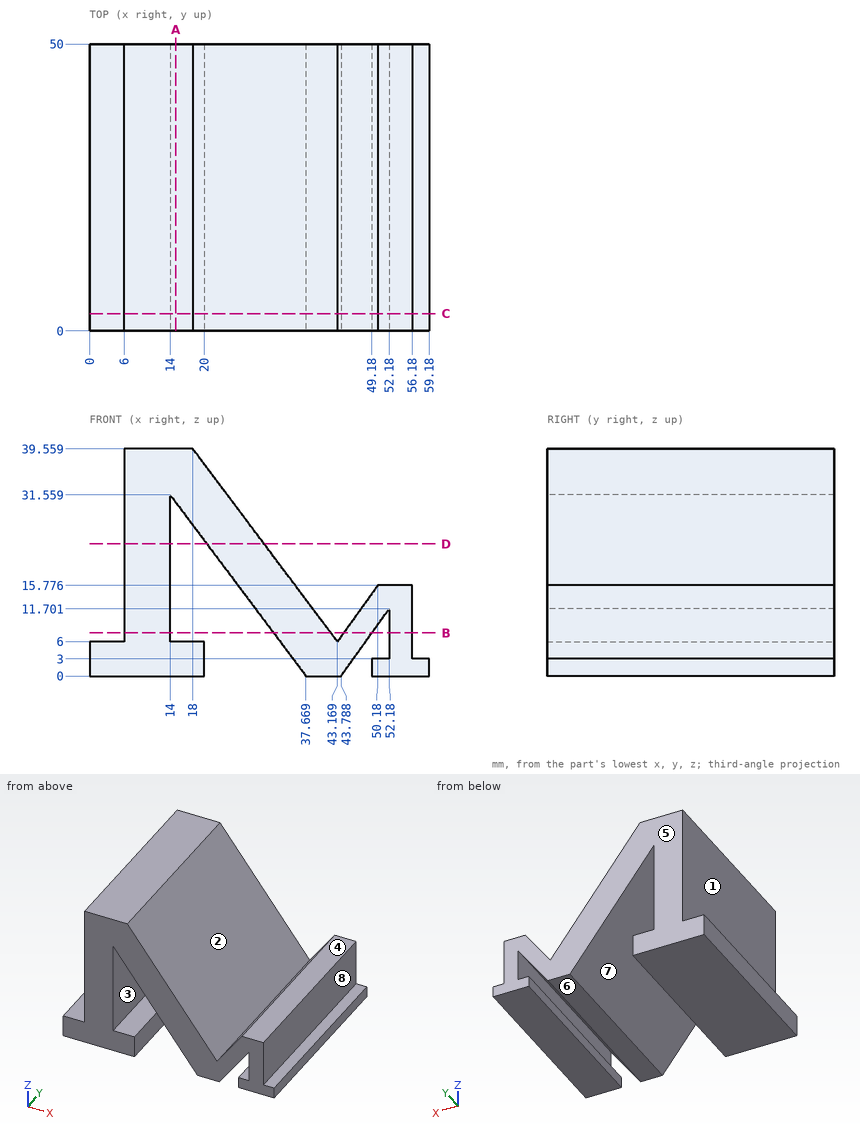
Can you work these out from the drawing? Everything is in mm from the part's minimum corner. A direction names the side the tool comes from. Give positions to 0.01 mm unless a question says otherwise; leave off trailing zeros. Write each loop counter-clockwise with the first axis right and the second up, starting at its lowest first coordinate (ties: lowest second). Pieces come first, ordered by that corner, then holes. Notation, with made-up numbers: (49, 8) -> (58, 8) arc R19 cw to (58, 25) -> close; hole circle Ø6 at (-27.75, -6). An arc over 180 degrees is marked (long way). Write each question's results on one line, items separated by ' | '. Start each with the question number.
Q1. We'd pull the mould along Z, two halves only. Please class the marked faces 6, 7 and 8: +Z half, -Z half, draft (parallel to the pull), parting line (faces both ways), or undercut.
Q2. I'm going to push flat-ended pins straight in: pin 1 Ø5 at (y, z) = (41.5, 31.5) entering from -X; pin 2 Ø5 at (x, y) = (54, 13.5) entering from +Z; pin 3 Ø5 at (x, y) = (1.5, 30) entering from +Z. Where does each tip first touch, or does it pass through?
Q3. Which directions (+Z, -Z, +X, -X, +Y, -Y) give clear straight access to the entire face, cutting with the end or side of a thin tool? Please do the marked faces 1, 2, 3, 4 and 5.
Q4. Suppose I cut it at B-B, the plane z = 7.5. List the corners of the cut face in (x, y) for me (1 decimal).
Q5. I need wall thicknesses on probe 1 along X at (y, z) = (41, 10.5) (1 decimal); probe 2 along X at (y, z) = (45, 10); probe 3 along X at (y, z) = (18, 5.5) (1 decimal). Which ranges of each line are inside material? Lowest first, please.
Q6. Suppose I cut it at D-D, the plane z = 23. List the corners of the cut face in (x, y) for me, and give its area (3 significant figures).
Q7. Suppose I cut it at C-C, the plane y = 3. List the corners of the cut face in (x, z) for me (1 decimal).
Q8. Suppose I cut it at A-A, the plane x = 15. List the corners of the cut face in (y, z) for me (1 decimal).
Outcome:
1) face 6: -Z half | face 7: undercut | face 8: draft
2) pin 1: x = 6 | pin 2: z = 15.78 | pin 3: z = 6
3) face 1: +Z, -X, +Y, -Y | face 2: +Z, +Y, -Y | face 3: +Y, -Y | face 4: +Z, +X, +Y, -Y | face 5: +Z, -Z, +X, -X, +Y
4) outline: (6, 0) -> (14, 0) -> (14, 50) -> (6, 50) -> close; (32, 0) -> (42, 0) -> (42, 50) -> (32, 50) -> close; (44.2, 0) -> (49.2, 0) -> (49.2, 50) -> (44.2, 50) -> close; (52.2, 0) -> (56.2, 0) -> (56.2, 50) -> (52.2, 50) -> close
5) probe 1: 6 to 14, 29.8 to 39.8, 46.4 to 51.3, 52.2 to 56.2 | probe 2: 6 to 14, 30.17 to 40.17, 46.04 to 50.96, 52.18 to 56.18 | probe 3: 0 to 20, 33.5 to 47.7, 52.2 to 56.2
6) outline: (6, 0) -> (14, 0) -> (14, 50) -> (6, 50) -> close; (20.42, 0) -> (30.42, 0) -> (30.42, 50) -> (20.42, 50) -> close | area: 900 mm2
7) outline: (0, 0) -> (20, 0) -> (20, 6) -> (14, 6) -> (14, 31.6) -> (37.7, 0) -> (43.8, 0) -> (52.2, 11.7) -> (52.2, 3) -> (49.2, 3) -> (49.2, 0) -> (59.2, 0) -> (59.2, 3) -> (56.2, 3) -> (56.2, 15.8) -> (50.2, 15.8) -> (43.2, 6) -> (18, 39.6) -> (6, 39.6) -> (6, 6) -> (0, 6) -> close
8) outline: (0, 0) -> (50, 0) -> (50, 6) -> (0, 6) -> close; (0, 30.2) -> (50, 30.2) -> (50, 39.6) -> (0, 39.6) -> close
